For this review, take the finished solid that the model builds, in its own axes (mm). Coordinates: 2 decimals unless noted, no trailing zeros. Loops run counter-clockwise (first coordinate to the right, second up) from the corner with the lowest first, then second, coordinate; pieces in that order, holes last. Notation, with made-up numbers: M 22,34 L 59,34 A36 cw 59,68 Z; hole C 45,28.25 d1. An arc over 180 degrees is marked long. Use one line per item in the form item = value.
Solid Edge part; units mm, degrees
sketch "Sketch1" plane through (0, 0, 0) normal (0, -1, 0) x (1, 0, 0)
  line L0 (-82.5, -82.5) -> (82.5, -82.5)
  line L1 (82.5, -82.5) -> (82.5, 82.5)
  line L2 (82.5, 82.5) -> (-82.5, 82.5)
  line L3 (-82.5, 82.5) -> (-82.5, -82.5)
  circle A0 centre (0, 0) radius 2
extrude "Protrusion1" add sketch "Sketch1" against normal blind 1
sketch "Sketch2" plane through (0, 0, 0) normal (0, -1, 0) x (1, 0, 0)
  circle A0 centre (0, 0) radius 8
extrude "Cutout1" cut sketch "Sketch2" against normal through all
sketch "Sketch3" plane through (0, 0, 0) normal (0, -1, 0) x (1, 0, 0)
  circle A0 centre (-75, 75) radius 2.5
  circle A1 centre (75, 75) radius 2.5
  circle A2 centre (75, -75) radius 2.5
  circle A3 centre (-75, -75) radius 2.5
extrude "Cutout2" cut sketch "Sketch3" against normal through all
sketch "Sketch4" plane through (0, 0, 0) normal (0, -1, 0) x (1, 0, 0)
  circle A0 centre (0, 11) radius 1.5
extrude "Cutout3" cut sketch "Sketch4" against normal through all
pattern_circular "Pattern1" count 6 over 360 about axis through (0, 0, 0) along (0, 1, 0) of "Cutout3"
properties material "Aluminum, 1060"
1. Wall thickness on line 1 along Z through (x, y) = (0, 0.4); line 2 along Z through (x, y) = (75, 0.5); line 3 along X through (y, z) = (0.85, -11): over which ranges is each line inside the solid? List them lowest first. Write a range as from..to.
Computed values:
line_1 = -82.5..-12.5, -9.5..-8, 8..9.5, 12.5..82.5
line_2 = -82.5..-77.5, -72.5..72.5, 77.5..82.5
line_3 = -82.5..-1.5, 1.5..82.5
2. Consider section C-C on z = 0. Write out the cut boundary in (x, y).
Computed values:
outline = M -82.5,0 L -8,0 L -8,1 L -82.5,1 Z; M 8,0 L 82.5,0 L 82.5,1 L 8,1 Z
3. Consider section B-B on z = -75. Write out the cut boundary in (x, y).
Computed values:
outline = M -82.5,0 L -77.5,0 L -77.5,1 L -82.5,1 Z; M -72.5,0 L 72.5,0 L 72.5,1 L -72.5,1 Z; M 77.5,0 L 82.5,0 L 82.5,1 L 77.5,1 Z
4. For pin 1 Ø6 at (x, z) = (-75, 75) entering from +Y, flat-tipped, find the tip position at first contact; note if it passes through.
Computed values:
pin_1 = 1
5. Draft analysis for pull direction Z (two halves, no side actions). For faces 1 (the face through (-77, 0.5, 73.5)), 2 (the face through (1, 1, -17)), state which applies: +Z half, -Z half, draft (parallel to the pull), parting line (faces both ways), or undercut.
Computed values:
face_1 = undercut
face_2 = draft
6. Consider section A-A on x = -75. Write out the cut boundary in (y, z).
Computed values:
outline = M 0,-82.5 L 1,-82.5 L 1,-77.5 L 0,-77.5 Z; M 0,-72.5 L 1,-72.5 L 1,72.5 L 0,72.5 Z; M 0,77.5 L 1,77.5 L 1,82.5 L 0,82.5 Z
